Model file for the job. Use its own axes, mm. A direction names the side the tool comes from. Coordinates: 2 decimals unless noted, no trailing zeros. Order: outer loops, then holes, each group sorted by start corner. A loop starts at its lowest first (then second) coordinate and runs counter-clockwise, first axis right, second up. Notation, with made-up numbers: (47, 73.5) -> (82, 73.5) arc R4 cw to (82, 78.5) -> close; hole circle Ø7 at (72.25, 36.5). An arc over 180 degrees is marked (long way). Return JSON: item names as keys, results as strings. Group by question number.
1) Cut at D-D (y = -3.75). Write the cut outline in (x, z), and give its area (3 significant figures).
2) Cut at A-A (y = 0). Write the cut outline in (x, z) (3 decimals), and give its area (3 significant figures).
3) Probe line 1 (X direction, y = 0, z = 5.45) (3 decimals); line 2 (Y direction, x = 0, z = 0.7) (3 decimals). List the from-to ranges inside material, lowest first.
4) Pull direction X, two halves, no side cores. Call faces 3 (the flat face through (1.2, -2.5, 2.54)), 4 (the cylindrical face through (-1.89, -1.45, 5.12)), 5 (the flat face through (6, 0, 0)), 6 (the cylindrical face through (12.719, 4.005, 4.85)): +X half, -X half, draft (parallel to the pull), parting line (faces both ways), or undercut.
5) Which spindle directions (+Z, -Z, +X, -X, +Y, -Y) get a long thin tool onto all of the face, cutting with end or side? Do faces 1 (the cylindrical face through (5.45, 1.72, 1.25)), 2 (the cylindrical face through (-0.19, 3.01, 7.85)). Say none if no direction does.
6) Flat gauge pins, fed straight in: pin 1 (1.5 mm diameter, centred on y = -9, z = 1.5, fed in from -X); pin 2 (1.5 mm diameter, centred on x = -4, y = 7.5, fed in from +Z); pin 3 (5 mm diameter, centred on x = -9.5, z = 8.5, fed in from +Y). Where does each tip first touch, or does it go through?
7) Cut at C-C (z = 1). Write the cut outline in (x, y) (3 decimals), and give its area (3 significant figures).
8) Cut at B-B (x = 0). Write the cut outline in (y, z) (3 decimals).
from build123d import *

# Parameters (mm, degrees)
F0_R          = 13.335
F0_R_2        = 5.715
F0_R_3        = 2.38125
F1_DEPTH      = 12.7
F2_DEPTH      = 2.54
F3_R          = 19.8268343705
F4_DEPTH      = 13.336
F4_DEPTH_BACK = 13.336


with BuildPart() as f1:
    # F0 (on Top) → F1 (new body)
    with BuildSketch(Plane.XY):
        Circle(F0_R)
        Circle(F0_R_2, mode=Mode.SUBTRACT)
        Circle(F0_R_2)
        Circle(F0_R_3, mode=Mode.SUBTRACT)
    extrude(amount=F1_DEPTH)

    # F0 (on Top) → F2 (cut)
    with BuildSketch(Plane.XY):
        Circle(F0_R_2)
        Circle(F0_R_3, mode=Mode.SUBTRACT)
    extrude(amount=F2_DEPTH, mode=Mode.SUBTRACT)

    # F3 (on Right) → F4 (cut, two sides)
    with BuildSketch(Plane.YZ) as f4_sk:
        with Locations((0, 27.4468343705)):
            Circle(F3_R)
    extrude(amount=-F4_DEPTH, mode=Mode.SUBTRACT)
    extrude(f4_sk.sketch, amount=F4_DEPTH_BACK, mode=Mode.SUBTRACT)


solid = f1.part
Answers below:
{
 "1": {"outline": "(-12.8, 0) -> (-4.31, 0) -> (-4.31, 2.54) -> (4.31, 2.54) -> (4.31, 0) -> (12.8, 0) -> (12.8, 7.98) -> (-12.8, 7.98) -> close", "area": "182 mm^2"},
 "2": {"outline": "(-13.335, 0) -> (-5.715, 0) -> (-5.715, 2.54) -> (-2.381, 2.54) -> (-2.381, 7.62) -> (-13.335, 7.62) -> close; (2.381, 2.54) -> (5.715, 2.54) -> (5.715, 0) -> (13.335, 0) -> (13.335, 7.62) -> (2.381, 7.62) -> close", "area": "150 mm^2"},
 "3": {"line 1": "x = -13.335 to -2.381, 2.381 to 13.335", "line 2": "y = -13.335 to -5.715, 5.715 to 13.335"},
 "4": {"face 3": "undercut", "face 4": "undercut", "face 5": "draft", "face 6": "parting line"},
 "5": {"face 1": "-Z", "face 2": "+Z, +X, -X"},
 "6": {"pin 1": "stops at x = -10.48", "pin 2": "stops at z = 9.42", "pin 3": "stops at y = 11.35"},
 "7": {"outline": "circle Ø26.67 at (0, 0); hole circle Ø11.43 at (0, 0)", "area": "456 mm^2"},
 "8": {"outline": "(-13.335, 0) -> (-5.715, 0) -> (-5.715, 2.54) -> (-2.381, 2.54) -> (-2.381, 7.764) arc R19.827 cw to (-13.253, 12.7) -> (-13.335, 12.7) -> close; (2.381, 2.54) -> (5.715, 2.54) -> (5.715, 0) -> (13.335, 0) -> (13.335, 12.7) -> (13.253, 12.7) arc R19.827 cw to (2.381, 7.764) -> close"}
}
